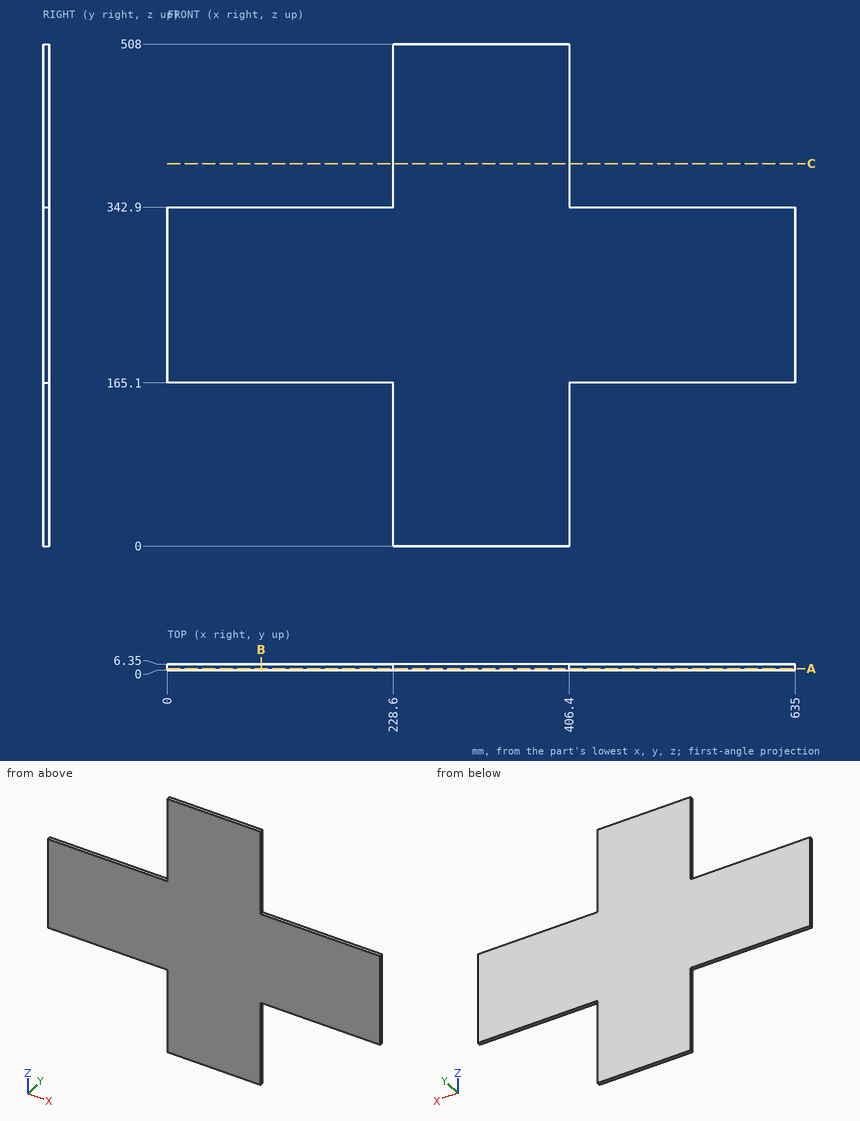
Verification items for this drawing (mm, ordinates from the low corner). Round coordinates to 2 decimals unless told otherwise and drop trailing zeros. Write each loop counter-clockwise with the first axis right and the second up, starting at its lowest first coordinate (ties: lowest second). Pieces come first, ordered by that corner, then holes. Notation, with made-up numbers: (1, -2.5) - (48, -2.5) arc R31 cw to (48, 21.5) - close; hole circle Ø4 at (51.5, -2.75). An arc over 180 degrees is marked (long way). Answer as a JSON object with one key per item and string values. Group by question number.
Q1. Go/stop test with flat-tipped pins: pin 1 Ø1.9 at (x, y) = (63, 2) entering from +Z; pin 2 Ø1.9 at (x, y) = (515.5, 3.5) entering from -Z; pin 3 Ø1.9 at (y, z) = (4, 449.5) entering from -X. Record where each tip stops, or that it passes through.
Q2. Thickness scan on line 1 (X direction, y = 1.25, z = 366); line 2 (Z direction, x = 149.5, y = 3.75). Record the ranges inside material, lowest first.
Q3. Section check C-C, the plane z = 387. Enter the section's corners in (x, y).
Q4. Section check A-A, the plane y = 1.75. Enter the section's corners in (x, z), plus the area to 3 significant figures.
Q5. Section check B-B, the plane x = 95. Enter the section's corners in (y, z), plus the area to 3 significant figures.
Found:
{
 "1": {"pin 1": "stops at z = 342.9", "pin 2": "stops at z = 165.1", "pin 3": "stops at x = 228.6"},
 "2": {"line 1": "x = 228.6 to 406.4", "line 2": "z = 165.1 to 342.9"},
 "3": {"outline": "(228.6, 0) - (406.4, 0) - (406.4, 6.35) - (228.6, 6.35) - close"},
 "4": {"outline": "(0, 165.1) - (228.6, 165.1) - (228.6, 0) - (406.4, 0) - (406.4, 165.1) - (635, 165.1) - (635, 342.9) - (406.4, 342.9) - (406.4, 508) - (228.6, 508) - (228.6, 342.9) - (0, 342.9) - close", "area": "172,000 mm^2"},
 "5": {"outline": "(0, 165.1) - (6.35, 165.1) - (6.35, 342.9) - (0, 342.9) - close", "area": "1,130 mm^2"}
}
